```python
from build123d import *

# Parameters (mm, degrees)
F0_R      = 5.4448713035
F1_DEPTH  = 46
F3_R      = 48.3631906875
F1_FACE_R = 5.4448713035
F5_T      = -2.5
F6_R      = 3.2055252898
F7_DEPTH  = 96.8010001


with BuildPart() as f1:
    # F0 (on Front) → F1 (new body)
    with BuildSketch(Plane.XZ):
        Circle(F0_R)
    extrude(amount=-F1_DEPTH)

    # F3 (on offset) → F4 section 0
    with BuildSketch(Plane.XZ.offset(50.8)):
        Circle(F3_R)
    # F1_face (on face) → F4 section 1
    with BuildSketch(Plane.XZ):
        Circle(F1_FACE_R)
    loft()

    # F5
    f5_openings = [f1.faces().sort_by_distance(p)[0] for p in [
        (0, -50.8, 0),
    ]]
    offset(amount=F5_T, openings=f5_openings, kind=Kind.INTERSECTION)

    # F6 (on face) → F7 (cut, through all)
    with BuildSketch(Plane(origin=(0, 46, 0), x_dir=(-1, 0, 0), z_dir=(0, 1, 0))):
        Circle(F6_R)
    extrude(amount=-F7_DEPTH, mode=Mode.SUBTRACT)


solid = f1.part
```
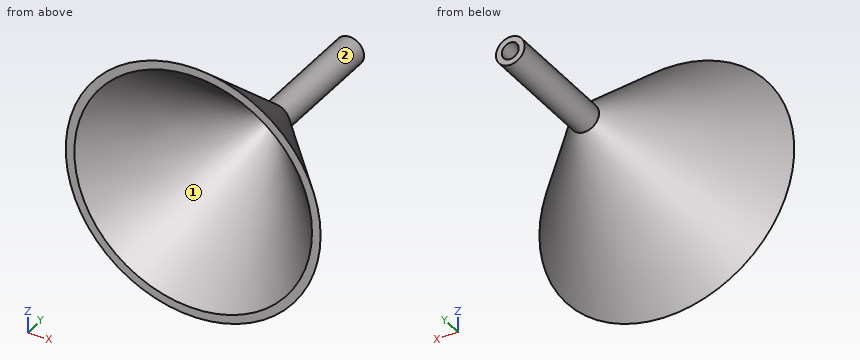
Build history of the part. All positions in model axes, mm. Face numbers are marked on the shaded views. Coordinates: 2 decimals unless noted, no trailing zeros. Order: outer loops, then holes, each group sorted by start corner. A loop starts at its lowest first (then second) coordinate and runs counter-clockwise, first axis right, second up.
Item 1: Drop flat-ended pins along their axis: pin 1 Ø3 at (x, z) = (-25, 2.5) entering from +Y; pin 2 Ø8.5 at (x, z) = (0, 0) entering from -Y; pin 3 Ø6 at (x, y) = (-11, -9) entering from -Z. Give the stop position or say it passes through.
Filled in:
pin 1: stops at y = -21.52
pin 2: stops at y = -2.46
pin 3: stops at z = -11.94
Item 2: Saw through at C-C on y = -43. List the corners of the cut face in (x, z), then the cut area to 3 significant figures.
Filled in:
outline: circle Ø83.55 at (0, 0); hole circle Ø77 at (0, 0)
area: 825 mm2
Item 3: Saw through at A-A on x = 0. List the corners of the cut face in (y, z).
Filled in:
outline: (-50.8, -48.36) - (0, -5.44) - (46, -5.44) - (46, -3.21) - (-1.22, -3.21) - (-50.8, -45.09) - close; (-50.8, 45.09) - (-1.22, 3.21) - (46, 3.21) - (46, 5.44) - (0, 5.44) - (-50.8, 48.36) - close
Item 4: Drill centre lines: L1, parallel to Z at x = 0, y = 24.5; L2, parallel to X at y = -37, z = 28; L3, parallel to X at y = 19, z = 2.5. Where is each one in solid material? Low to high.
Filled in:
L1: z = -5.44 to -3.21, 3.21 to 5.44
L2: x = -23.73 to -18.27, 18.27 to 23.73
L3: x = -4.84 to -2.01, 2.01 to 4.84
Item 5: Mould opens along X. For the marked faces 1 and 2 say: released by +X, released by -X, zero draft, split by the parting line, or undercut.
Filled in:
face 1: undercut
face 2: split by the parting line
Item 6: Saw through at B-B on y = 17.5. List the corners of the cut face in (x, z), then the cut area to 3 significant figures.
Filled in:
outline: circle Ø10.89 at (0, 0); hole circle Ø6.41 at (0, 0)
area: 60.9 mm2
